Can you work these out from the model? Positions are in its coordinate system, mm. Coordinates: 2 decimals unless noted, no trailing zeros. Order: outer loops, then holes, each group sorted by start corner. A loop starts at its lowest first (then second) coordinate and runs counter-clockwise, first axis right, second up. Notation, with made-up numbers: (51.25, 85) -> (91.25, 85) arc R23 ccw to (91.25, 94) -> close; hole circle Ø4 at (25.5, 54.5). An arc over 180 degrees is marked (long way). Write item = value, one per line.
```python
from build123d import *

# Parameters (mm, degrees)
BASE_EXTRUDE_DEPTH = 3.175
SKETCH3_R          = 9.525
SKETCH3_R_2        = 10
SKETCH3_R_3        = 7.9375
HOLES_DEPTH        = 4.175


with BuildPart() as part:
    # Sketch2 → Base Extrude (new body)
    with BuildSketch(Plane.XY):
        Polygon((0, 0), (100, 0), (100, 30), (167.901300028, 86.97595581), (169.276751583, 102.697439025), (159.132575314, 114.786797538), (143.411092099, 116.162249093), (71.118715891, 55.50174288), (56.435934796, 73), (6.435934796, 73), (0, 36.5), align=None)
    extrude(amount=BASE_EXTRUDE_DEPTH)

    # Sketch3 → Holes (cut, through all)
    with BuildSketch(Plane.XY.offset(3.175)):
        with Locations((150.882386677, 97.563400756)):
            Circle(SKETCH3_R)
        with Locations((127.901053383, 78.279772465)):
            Circle(SKETCH3_R)
        with Locations((104.91972009, 58.996144175)):
            Circle(SKETCH3_R_2)
        with Locations((30.39150811, 52.766671577)):
            Circle(SKETCH3_R_3)
        with Locations((50.39150811, 52.766671577)):
            Circle(SKETCH3_R_3)
        with Locations((10.39150811, 32.766671577)):
            Circle(SKETCH3_R_3)
        with Locations((30.39150811, 32.766671577)):
            Circle(SKETCH3_R_3)
        with Locations((50.39150811, 32.766671577)):
            Circle(SKETCH3_R_3)
        with Locations((70.39150811, 32.766671577)):
            Circle(SKETCH3_R_3)
        with Locations((30.39150811, 12.766671577)):
            Circle(SKETCH3_R_3)
        with Locations((50.39150811, 12.766671577)):
            Circle(SKETCH3_R_3)
        with Locations((70.39150811, 12.766671577)):
            Circle(SKETCH3_R_3)
        with Locations((90.39150811, 32.766671577)):
            Circle(SKETCH3_R_3)
    extrude(amount=-HOLES_DEPTH, mode=Mode.SUBTRACT)


solid = part.part
```
Item 1: I want a section at B-B, the plane y = 99.5. Please give me the cut outline in (x, z) (3 decimals).
A:
outline = (123.554, 0) -> (141.556, 0) -> (141.556, 3.175) -> (123.554, 3.175) -> close; (160.208, 0) -> (168.997, 0) -> (168.997, 3.175) -> (160.208, 3.175) -> close
Item 2: I want a section at A-A, the plane x = 36.5. Please give me the cut outline in (y, z) (3 decimals), plus the area to 3 significant figures.
A:
outline = (0, 0) -> (7.698, 0) -> (7.698, 3.175) -> (0, 3.175) -> close; (17.835, 0) -> (27.698, 0) -> (27.698, 3.175) -> (17.835, 3.175) -> close; (37.835, 0) -> (47.698, 0) -> (47.698, 3.175) -> (37.835, 3.175) -> close; (57.835, 0) -> (73, 0) -> (73, 3.175) -> (57.835, 3.175) -> close
area = 135 mm2
Item 3: I want a section at C-C, the plane x = 122.5. Please give me the cut outline in (y, z) (3 decimals).
A:
outline = (48.88, 0) -> (70.434, 0) -> (70.434, 3.175) -> (48.88, 3.175) -> close; (86.125, 0) -> (98.616, 0) -> (98.616, 3.175) -> (86.125, 3.175) -> close
Item 4: If I drill on probe 1 along Y at (x, z) = (51, 2.7); probe 2 along X at (y, z) = (27, 0.75); probe 3 along X at (y, z) = (28.5, 1.1), over which ranges is the centre line in solid material (lowest first)?
A:
probe_1 = 0 to 4.85, 20.68 to 24.85, 40.68 to 44.85, 60.68 to 73
probe_2 = 0 to 4.94, 15.85 to 24.94, 35.85 to 44.94, 55.85 to 64.94, 75.85 to 84.94, 95.85 to 100
probe_3 = 0 to 3.7, 17.08 to 23.7, 37.08 to 43.7, 57.08 to 63.7, 77.08 to 83.7, 97.08 to 100
Item 5: If we mould it in two halves opening along Y, with no side actions, what happens to faces 1 (the flat face through (100, 15, 2)), 2 (the cylindrical face through (62.46, 13.12, 1.61)), 3 (the flat face through (168.58, 94.73, 1.57)), 4 (the flat face through (63.88, 64.13, 1.57))? For each: pulls with the +Y half, pulls with the -Y half, needs draft (parallel to the pull), parting line crosses it, or undercut.
A:
face_1 = needs draft
face_2 = undercut
face_3 = pulls with the -Y half
face_4 = pulls with the +Y half
Item 6: I'm going to push flat-ended pins straight in: P1, Ø1, axis at y = 55, z = 1.5, coming from the -X side; P2, Ø1.6, axis at y = 17.5, z = 1.5, coming from the +X side; P3, Ø1.5, axis at x = 106.5, z = 2, coming from the +Y side. Where does each tip first touch, or does it pass through?
A:
P1 = 3.17
P2 = 100
P3 = 85.82
Item 7: I want a section at D-D, the plane z = 2. Give the number of separate pieces and of enclosed holes in the cut face, plus the area to 3 significant figures.
A:
separate_pieces = 1
enclosed_holes = 13
area = 7,100 mm2
